Check sheet for the drawn part. Datum: minimum x, y, z corner. Units: mm. A direction names the side the tool comes from. Coordinates: 2 decimals unless noted, no trailing zeros. Write each loop counter-clockwise with the first axis right and the second up, starting at its lowest first coordinate (ties: lowest second). Pieces come first, ordered by that corner, then holes. Notation, with made-up numbers: (-33.75, -36.75) -> (3.25, -36.75) arc R23 cw to (3.25, -8.75) -> close; hole circle Ø5 at (59, 29.25). An arc over 180 degrees is marked (long way). Answer in a Markdown table with one row per item.
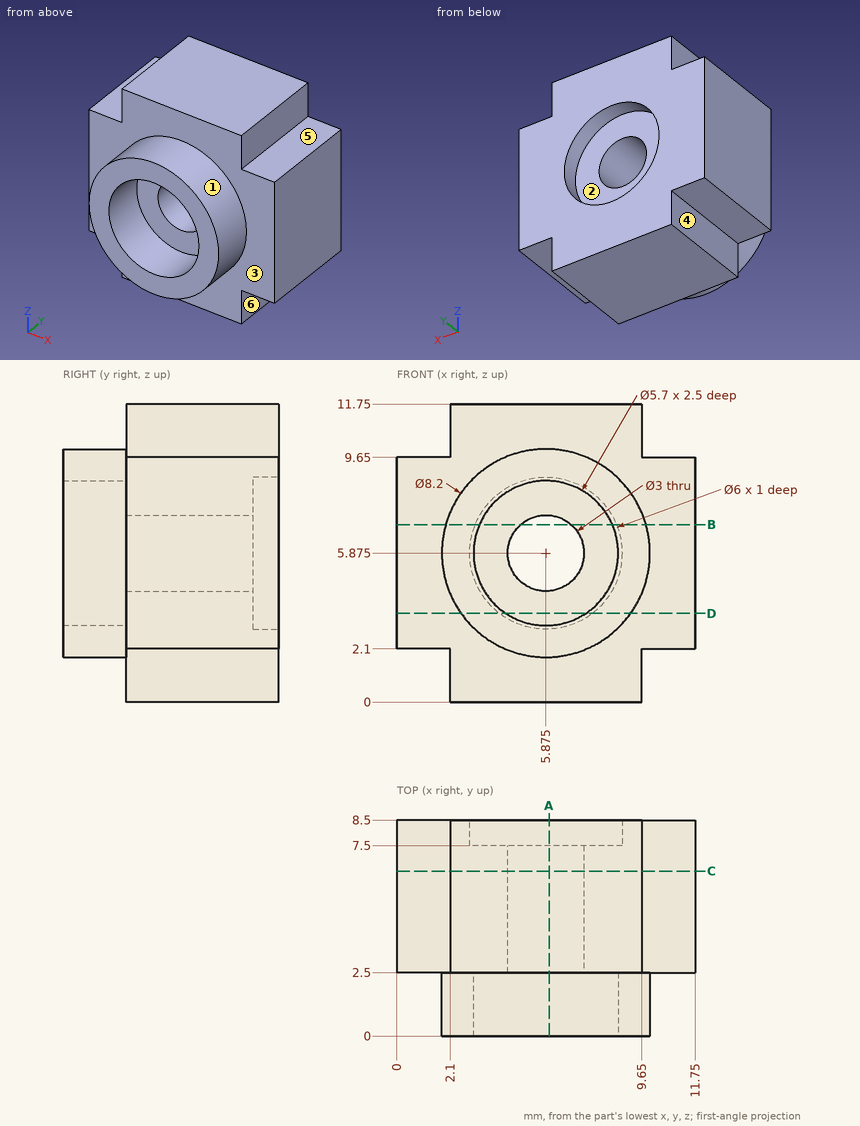
1. Material ranges on probe 1 along X at (y, z) = (6, 1.5); probe 2 along Y at (x, z) = (3.5, 5), recorded low to high. Write a range as from..to.
Findings below:
| item | result |
|---|---|
| probe 1 | x = 2.1..9.65 |
| probe 2 | y = 2.5..7.5 |
2. Sectioned sample at D-D, the plane z = 3.5. Record the cut outline in (x, y), and give its area (3 significant figures).
Findings below:
| item | result |
|---|---|
| outline | (0, 2.5) -> (2.53, 2.5) -> (2.53, 0) -> (4.3, 0) -> (4.3, 2.5) -> (7.45, 2.5) -> (7.45, 0) -> (9.22, 0) -> (9.22, 2.5) -> (11.75, 2.5) -> (11.75, 8.5) -> (7.71, 8.5) -> (7.71, 7.5) -> (4.04, 7.5) -> (4.04, 8.5) -> (0, 8.5) -> close |
| area | 75.7 mm² |
3. Sectioned sample at C-C, the plane y = 6.5. Record the cut outline in (x, z) (3 decimals).
Findings below:
| item | result |
|---|---|
| outline | (0, 2.1) -> (2.1, 2.1) -> (2.1, 0) -> (9.65, 0) -> (9.65, 2.1) -> (11.75, 2.1) -> (11.75, 9.65) -> (9.65, 9.65) -> (9.65, 11.75) -> (2.1, 11.75) -> (2.1, 9.65) -> (0, 9.65) -> close; hole circle Ø3 at (5.875, 5.875) |
4. Go/stop test with flat-tipped pins: pin 1 (0.6 mm diameter, centred on y = 5.5, z = 10.5, fed in from +X); pin 2 (3.5 mm diameter, centred on x = 5.875, z = 5.875, fed in from +Y); pin 3 (0.6 mm diameter, centred on x = 11, y = 6, fed in from +Z). Record where each tip stops, or that it passes through.
Findings below:
| item | result |
|---|---|
| pin 1 | stops at x = 9.65 |
| pin 2 | stops at y = 7.5 |
| pin 3 | stops at z = 9.65 |
5. Access from +Z, -Z, +X, -X, +Y, -Y to the whole of each face (thin tool, end or side, straight path). Record for the marked faces 4, 5 and 6.
Findings below:
| item | result |
|---|---|
| face 4 | -Z, -X, +Y, -Y |
| face 5 | +Z, +X, +Y, -Y |
| face 6 | -Z, +X, +Y, -Y |
6. Sectioned sample at A-A, the plane x = 6. Record the cut outline in (y, z).
Findings below:
| item | result |
|---|---|
| outline | (0, 1.78) -> (2.5, 1.78) -> (2.5, 0) -> (8.5, 0) -> (8.5, 2.88) -> (7.5, 2.88) -> (7.5, 4.38) -> (2.5, 4.38) -> (2.5, 3.03) -> (0, 3.03) -> close; (0, 8.72) -> (2.5, 8.72) -> (2.5, 7.37) -> (7.5, 7.37) -> (7.5, 8.87) -> (8.5, 8.87) -> (8.5, 11.75) -> (2.5, 11.75) -> (2.5, 9.97) -> (0, 9.97) -> close |
7. Release check for a two-part mould opening along X. For the marked faces 1, 2 and 3 record: released by +X, released by -X, zero draft, split by the parting line, or undercut.
Findings below:
| item | result |
|---|---|
| face 1 | split by the parting line |
| face 2 | undercut |
| face 3 | zero draft |
8. Sectioned sample at B-B, the plane z = 7. Record the cut outline in (x, y), and give its area (3 significant figures).
Findings below:
| item | result |
|---|---|
| outline | (0, 2.5) -> (1.93, 2.5) -> (1.93, 0) -> (3.26, 0) -> (3.26, 2.5) -> (4.88, 2.5) -> (4.88, 7.5) -> (3.09, 7.5) -> (3.09, 8.5) -> (0, 8.5) -> close; (6.87, 2.5) -> (8.49, 2.5) -> (8.49, 0) -> (9.82, 0) -> (9.82, 2.5) -> (11.75, 2.5) -> (11.75, 8.5) -> (8.66, 8.5) -> (8.66, 7.5) -> (6.87, 7.5) -> close |
| area | 61.6 mm² |
